from build123d import *

# Parameters (mm, degrees)
F0_R     = 4.7625
F1_DEPTH = 25.4


with BuildPart() as f1:
    # F0 (on Top) → F1 (new body)
    with BuildSketch(Plane.XY):
        Polygon((-219.075, 165.1), (-219.075, 19.05), (-200.787, 19.05), (-128.5875, 91.2495), (-146.9525612107, 109.6145612107), (-202.438, 165.1), align=None)
        Polygon((-38.1, 0.762), (-38.1, 19.05), (-200.787, 19.05), (-219.075, 0.762), align=None)
        with Locations((-203.2, 9.525)):
            Circle(F0_R, mode=Mode.SUBTRACT)
        with Locations((-177.8, 9.525)):
            Circle(F0_R, mode=Mode.SUBTRACT)
        with Locations((-152.4, 9.525)):
            Circle(F0_R, mode=Mode.SUBTRACT)
        with Locations((-127, 9.525)):
            Circle(F0_R, mode=Mode.SUBTRACT)
        with Locations((-101.6, 9.525)):
            Circle(F0_R, mode=Mode.SUBTRACT)
        with Locations((-76.2, 9.525)):
            Circle(F0_R, mode=Mode.SUBTRACT)
        with Locations((-50.8, 9.525)):
            Circle(F0_R, mode=Mode.SUBTRACT)
        with BuildLine():
            Line((-125.1955164365, 94.6414835635), (-128.5875, 91.2495))
            Line((-128.5875, 91.2495), (-57.15, 19.812))
            Line((-57.15, 19.812), (-44.3645546077, 32.5974453923))
            Line((-44.3645546077, 32.5974453923), (-115.8020546077, 104.0349453923))
            Line((-115.8020546077, 104.0349453923), (-118.5090993819, 101.3279006181))
            ThreePointArc((-118.5090993819, 101.3279006181), (-117.7551848926, 99.9437041782), (-117.4943568778, 98.3892410594))
            ThreePointArc((-117.4943568778, 98.3892410594), (-120.1728655028, 94.1069068595), (-125.1955164365, 94.6414835635))
        make_face()
        with Locations((-68.3753201513, 44.5077043329)):
            Circle(F0_R, mode=Mode.SUBTRACT)
        with Locations((-86.3358323935, 62.4682165751)):
            Circle(F0_R, mode=Mode.SUBTRACT)
        with Locations((-104.2963446356, 80.4287288172)):
            Circle(F0_R, mode=Mode.SUBTRACT)
        Polygon((-200.787, 19.05), (-219.075, 19.05), (-219.075, 0.762), align=None)
        with BuildLine():
            Line((-176.8671092154, 165.1), (-202.438, 165.1))
            Line((-202.438, 165.1), (-146.9525612107, 109.6145612107))
            Line((-146.9525612107, 109.6145612107), (-143.5849651653, 112.9821572561))
            ThreePointArc((-143.5849651653, 112.9821572561), (-143.5849651653, 119.7173493469), (-136.8497730745, 119.7173493469))
            Line((-136.8497730745, 119.7173493469), (-134.1671158184, 122.400006603))
            Line((-134.1671158184, 122.400006603), (-176.8671092154, 165.1))
        make_face()
        with Locations((-158.177881362, 134.3102655436)):
            Circle(F0_R, mode=Mode.SUBTRACT)
        with Locations((-176.1383936042, 152.2707777858)):
            Circle(F0_R, mode=Mode.SUBTRACT)
        with BuildLine():
            Line((-146.9525612107, 109.6145612107), (-128.5875, 91.2495))
            Line((-128.5875, 91.2495), (-125.1955164365, 94.6414835635))
            ThreePointArc((-125.1955164365, 94.6414835635), (-125.6244529232, 101.7568371048), (-118.5090993819, 101.3279006181))
            Line((-118.5090993819, 101.3279006181), (-115.8020546077, 104.0349453923))
            Line((-115.8020546077, 104.0349453923), (-134.1671158184, 122.400006603))
            Line((-134.1671158184, 122.400006603), (-136.8497730745, 119.7173493469))
            ThreePointArc((-136.8497730745, 119.7173493469), (-135.8173928463, 118.1722831481), (-135.4548691199, 116.3497533015))
            ThreePointArc((-135.4548691199, 116.3497533015), (-138.3948392733, 111.9497770279), (-143.5849651653, 112.9821572561))
            Line((-143.5849651653, 112.9821572561), (-146.9525612107, 109.6145612107))
        make_face()
        Polygon((-200.787, 19.05), (-38.1, 19.05), (-38.1, 26.3328907846), (-44.3645546077, 32.5974453923), (-57.15, 19.812), (-128.5875, 91.2495), align=None)
    extrude(amount=F1_DEPTH)


solid = f1.part
Input: part model. Units: mm. Frame: model coordinates. Coordinates: 2 decimals unless noted, no trailing zeros. Order: outer loops, then holes, each group sorted by start corner. A loop starts at its lowest first (then second) coordinate and runs counter-clockwise, first axis right, second up. Notation, with made-up numbers: M 70,46 L 80,46 A10 ccw 80,61 Z; hole C -13,27 d11. An arc over 180 degrees is marked long. Answer as CSV lines item,"result".
1. Material intervals for line 1 (Y direction, x = -179.5, z = 8.75); line 2 (Y direction, x = -155, z = 13); line 3 (X direction, y = 152, z = 2) (3 decimals), sorted ascending. Write a range as from..to.
Reported:
line 1,"0.76..5.08, 13.97..148.9, 155.64..165.1"
line 2,"0.76..5.53, 13.52..130.76, 137.86..143.23"
line 3,"-219.075..-180.893, -171.384..-163.767"
2. Section C-C (x = -101.6). Return the cut outline in (y, z), then the cut area to 3 significant figures.
Reported:
outline,"M 0.76,0 L 4.76,0 L 4.76,25.4 L 0.76,25.4 Z; M 14.29,0 L 76.5,0 L 76.5,25.4 L 14.29,25.4 Z; M 84.35,0 L 89.83,0 L 89.83,25.4 L 84.35,25.4 Z"
area,"1,820 mm2"
3. Section D-D (x = -53.5). Return the cut outline in (y, z), then the cut area to 3 significant figures.
Reported:
outline,"M 0.76,0 L 5.6,0 L 5.6,25.4 L 0.76,25.4 Z; M 13.45,0 L 41.73,0 L 41.73,25.4 L 13.45,25.4 Z"
area,"841 mm2"
4. Section B-B (z = 13.5). State how many separate pieces and enclosed holes the cut face has, then the cut area to 3 significant figures.
Reported:
separate pieces,"1"
enclosed holes,"14"
area,"19,100 mm2"
5. Pull-direction query (Y, two-part tool) for faces 1 (the flat face through (-130, 0.762, 13)), 2 (the flat face through (-106.512, 94.745, 12.522)), 3 (the cylindrical face through (-54.58, 6.63, 12.52)), 4 (the flat face through (-150, 66, 25.4)); classes: released by +Y, released by -Y, zero draft, split by the parting line, or undercut.
Reported:
face 1,"released by -Y"
face 2,"released by +Y"
face 3,"undercut"
face 4,"zero draft"
6. First-contact query: P1, Ø6, axis at y = 127, z = 12.5, coming from the +X side; P2, Ø7.5, axis at x = -127, y = 9.525, coming from the -Z side; P3, Ø5, axis at x = -83.5, z = 8.5, coming from the +Y side; P4, Ø2, axis at x = -75.5, z = 7, coming from the +Y side. Flat tips, straight axial feed; report the tip coordinate or a pass-through.
Reported:
P1,"x = -135.77"
P2,"through"
P3,"y = 74.23"
P4,"y = 64.73"
7. Section A-A (x = -203.2). Return the cut outline in (y, z).
Reported:
outline,"M 0.76,0 L 4.76,0 L 4.76,25.4 L 0.76,25.4 Z; M 14.29,0 L 165.1,0 L 165.1,25.4 L 14.29,25.4 Z"
